Answer from the drawing. Dimensions are ordinates in mm from the lowest x, y and z of the part. Coordinates: 2 decimals unless noted, no trailing zeros. Order: outer loops, then holes, each group sorted by start corner. A loop starts at its lowest first (then second) coordinate and runs counter-clockwise, first axis right, second up. Notation, with made-up numbers: (26, 23) -> (34, 23) arc R29 cw to (34, 55) -> close; hole circle Ø4 at (54.5, 36). An arc over 180 degrees is marked (long way). Use CSV: the item, a comma, the result in double quotes.
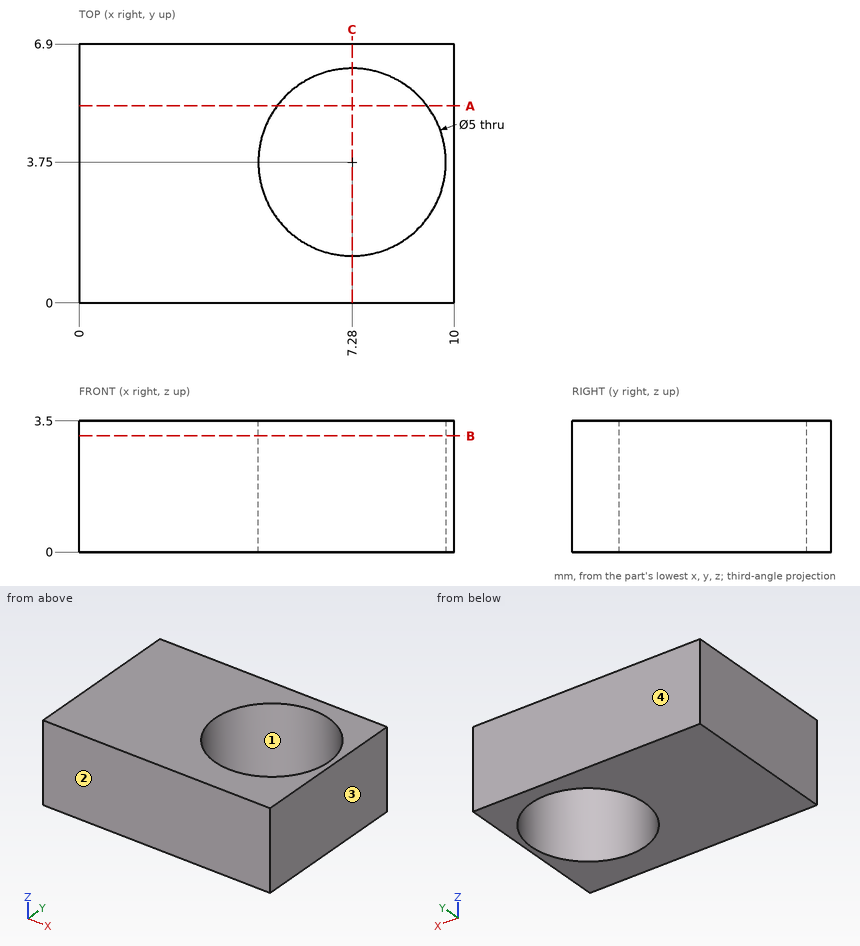
Item 1: This flat-tipped pin is pushed along its axis until it touches: P1, Ø2, axis at x = 4.5, z = 2, coming from the -Y side. Where does it stop, or does it pass through?
Return value:
P1,"stops at y = 0"
Item 2: Straight lines are drawn through the part: line 1 along Y through (x, z) = (7.28, 2.05); line 2 along Y through (x, z) = (5, 0.45); line 3 along X through (y, z) = (3.25, 1.7). For each, find the intervals that lie inside material, in ascending order.
Return value:
line 1,"y = 0 to 1.25, 6.25 to 6.9"
line 2,"y = 0 to 2.72, 4.78 to 6.9"
line 3,"x = 0 to 4.83, 9.73 to 10"
Item 3: Find section C-C, the plane x = 7.28. Give the vertices of the cut face in (y, z), then the cut area to 3 significant figures.
Return value:
outline,"(0, 0) -> (1.25, 0) -> (1.25, 3.5) -> (0, 3.5) -> close; (6.25, 0) -> (6.9, 0) -> (6.9, 3.5) -> (6.25, 3.5) -> close"
area,"6.65 mm^2"
Item 4: The mould has two halves that part along Y. Classify the marked faces 1, 2, 3 and 4: +Y half, -Y half, draft (parallel to the pull), parting line (faces both ways), or undercut.
Return value:
face 1,"undercut"
face 2,"-Y half"
face 3,"draft"
face 4,"+Y half"
Item 5: Find section A-A, the plane y = 5.25. Give the vertices of the cut face in (x, z).
Return value:
outline,"(0, 0) -> (5.28, 0) -> (5.28, 3.5) -> (0, 3.5) -> close; (9.28, 0) -> (10, 0) -> (10, 3.5) -> (9.28, 3.5) -> close"
Item 6: Find section B-B, the plane z = 3.1. Give the vertices of the cut face in (x, y).
Return value:
outline,"(0, 0) -> (10, 0) -> (10, 6.9) -> (0, 6.9) -> close; hole circle Ø5 at (7.28, 3.75)"
